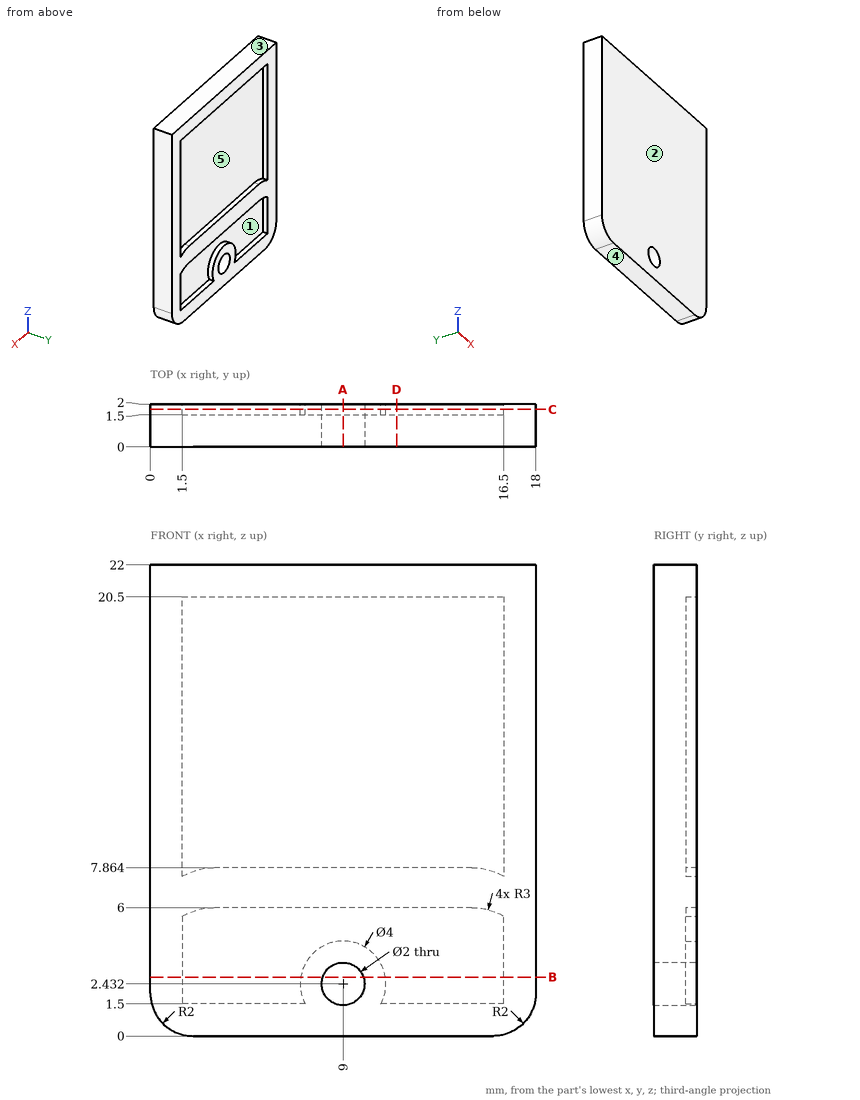
Geometry check sheet. Reference: drawing and pictorial views, mm from the part's lowest x, y, z. A direction names the side the tool comes from. Give positions to 0.01 mm unless a question says otherwise; leave off trailing zeros. Write each loop counter-clockwise with the first axis right and the second up, starting at its lowest first coordinate (ties: lowest second). Pieces come first, ordered by that corner, then holes. Notation, with made-up numbers: (39.5, 87.5) - (45.5, 87.5) arc R18 cw to (45.5, 110.5) - close; hole circle Ø11 at (-19, 56.5). An arc over 180 degrees is marked (long way). Put each result on its own line as item: value.
Q1. Section check B-B on z = 2.75. Record the cut outline in (x, y).
Result:
outline: (0, 0) - (8.05, 0) - (8.05, 2) - (7.03, 2) - (7.03, 1.5) - (1.5, 1.5) - (1.5, 2) - (0, 2) - close; (9.95, 0) - (18, 0) - (18, 2) - (16.5, 2) - (16.5, 1.5) - (10.97, 1.5) - (10.97, 2) - (9.95, 2) - close
Q2. Section check A-A on x = 9. Record the cut outline in (y, z).
Result:
outline: (0, 0) - (2, 0) - (2, 1.43) - (0, 1.43) - close; (0, 3.43) - (2, 3.43) - (2, 4.43) - (1.5, 4.43) - (1.5, 6) - (2, 6) - (2, 7.86) - (1.5, 7.86) - (1.5, 20.5) - (2, 20.5) - (2, 22) - (0, 22) - close
Q3. Set-up check for the marked faces 1 and 2: record each of +Z, -Z, +X, -X, +Y, -Y from which the full face is reachable in a straight line by a thin tool's end or side.
Result:
face 1: +Y
face 2: +Z, -Z, +X, -X, -Y
Q4. Mould release check, pull along Z, two halves, no side actions. Record for the marked faces 3, 4 and 5: released by +Z, released by -Z, zero draft, split by the parting line, or undercut.
Result:
face 3: released by +Z
face 4: released by -Z
face 5: undercut
Q5. Section check C-C on y = 1.75. Record the cut outline in (x, z), and give its area (3 significant figures).
Result:
outline: (0, 2) arc R2 ccw to (2, 0) - (16, 0) arc R2 ccw to (18, 2) - (18, 22) - (0, 22) - close; hole (1.5, 1.5) - (7.23, 1.5) arc R2 cw (long way) to (10.77, 1.5) - (16.5, 1.5) - (16.5, 5.6) arc R3 ccw to (15, 6) - (3, 6) arc R3 ccw to (1.5, 5.6) - close; hole (1.5, 7.46) arc R3 cw to (3, 7.86) - (15, 7.86) arc R3 cw to (16.5, 7.46) - (16.5, 20.5) - (1.5, 20.5) - close; hole circle Ø2 at (9, 2.43)
area: 144 mm2
Q6. Section check D-D on x = 11.5. Record the cut outline in (y, z), and give its area (3 significant figures).
Result:
outline: (0, 0) - (2, 0) - (2, 1.5) - (1.5, 1.5) - (1.5, 6) - (2, 6) - (2, 7.86) - (1.5, 7.86) - (1.5, 20.5) - (2, 20.5) - (2, 22) - (0, 22) - close
area: 35.4 mm2
Q7. Scan lines: probe 1 along Z at (x, y) = (13.75, 1.95); probe 2 along Z at (x, y) = (9, 0.75); probe 3 along X at (y, z) = (1.75, 18.5). Record each from-to range of solid material in increasing order. Write a range as from..to.
Result:
probe 1: 0..1.5, 6..7.86, 20.5..22
probe 2: 0..1.43, 3.43..22
probe 3: 0..1.5, 16.5..18
